from build123d import *

# Parameters (mm, degrees)
BOSS_EXTRUDE3_DEPTH = 12
BOSS_EXTRUDE4_DEPTH = 20
BOSS_EXTRUDE5_DEPTH = 12
SKETCH12_W          = 16
SKETCH12_H          = 40
CUT_EXTRUDE1_DEPTH  = 96.833188406
SKETCH13_R          = 8
CUT_EXTRUDE2_DEPTH  = 94.808315196
SKETCH14_R          = 8
CUT_EXTRUDE3_DEPTH  = 96.833188406
SKETCH15_R          = 8
CUT_EXTRUDE4_DEPTH  = 119.321595662
FILLET1_R           = 3
FILLET2_R           = 2


with BuildPart() as part:
    # Sketch7 → Boss-Extrude3 (new body)
    with BuildSketch(Plane(origin=(0, 0, 0), x_dir=(0, 1, 0), z_dir=(0, 0, 1))):
        with BuildLine():
            Line((0, -20), (0, 20))
            Line((0, 20), (40, 20))
            ThreePointArc((40, 20), (60, 0), (40, -20))
            Line((40, -20), (0, -20))
        make_face()
    extrude(amount=BOSS_EXTRUDE3_DEPTH)

    # Sketch9 → Boss-Extrude4 (add, symmetric)
    with BuildSketch(Plane.YZ):
        with BuildLine():
            Line((0, 0), (-40, 0))
            Line((-40, 0), (-40, 40))
            ThreePointArc((-40, 40), (-20, 60), (0, 40))
            Line((0, 40), (0, 0))
        make_face()
    extrude(amount=BOSS_EXTRUDE4_DEPTH, both=True)

    # Sketch10 → Boss-Extrude5 (add)
    with BuildSketch(Plane.XZ.offset(40)):
        with BuildLine():
            Line((-20, 0), (20, 0))
            Line((20, 0), (20, -39.999997874))
            ThreePointArc((20, -39.999997874), (1.063e-06, -60), (-20, -40))
            Line((-20, -40), (-20, 0))
        make_face()
    extrude(amount=-BOSS_EXTRUDE5_DEPTH)

    # Sketch12 → Cut-Extrude1 (cut, through all)
    with BuildSketch(Plane.XY.offset(12)):
        with Locations((0, -20)):
            Rectangle(SKETCH12_W, SKETCH12_H)
    extrude(amount=CUT_EXTRUDE1_DEPTH, mode=Mode.SUBTRACT)

    # Sketch13 → Cut-Extrude2 (cut, through all)
    with BuildSketch(Plane.YZ.offset(20)):
        with Locations((-20, 40)):
            Circle(SKETCH13_R)
    extrude(amount=-CUT_EXTRUDE2_DEPTH, mode=Mode.SUBTRACT)

    # Sketch14 → Cut-Extrude3 (cut, through all)
    with BuildSketch(Plane.XY.offset(12)):
        with Locations((0, 40)):
            Circle(SKETCH14_R)
    extrude(amount=-CUT_EXTRUDE3_DEPTH, mode=Mode.SUBTRACT)

    # Sketch15 → Cut-Extrude4 (cut, through all)
    with BuildSketch(Plane.XZ.offset(40)):
        with Locations(Location((0, -40, 0), (0, 0, 270))):
            Circle(SKETCH15_R)
    extrude(amount=-CUT_EXTRUDE4_DEPTH, mode=Mode.SUBTRACT)

    # Fillet1
    fillet1_edges = [part.edges().sort_by_distance(p)[0] for p in [
        (14, 0, 12),
        (-14, 0, 12),
    ]]
    fillet(fillet1_edges, radius=FILLET1_R)

    # Fillet2
    fillet2_edges = [part.edges().sort_by_distance(p)[0] for p in [
        (0, -28, 0),
    ]]
    fillet(fillet2_edges, radius=FILLET2_R)


solid = part.part
Here's how the part is built. I have some questions about the finished solid (model axes, mm). A direction names the side the tool comes from. Round coordinates to 2 decimals unless told otherwise and drop trailing zeros. Order: outer loops, then holes, each group sorted by start corner. A loop starts at its lowest first (then second) coordinate and runs counter-clockwise, first axis right, second up. Notation, with made-up numbers: (-17.75, -2.75) -> (41.25, -2.75) arc R22 cw to (41.25, 8.25) -> close; hole circle Ø3 at (27.5, 8.25). An arc over 180 degrees is marked (long way). Return JSON: item names as keys, results as strings.
Q1. For pin 1 Ø20 at (x, y) = (-7.5, 6) entering from +Z; pin 2 Ø1 at (x, y) = (10.5, 40.5) entering from -Z; pin 3 Ø1.5 at (x, z) = (0.5, -47) entering from +Y; pin 4 Ø1.5 at (x, z) = (-6.5, -36) entering from +Y, each with a flat end and sliding along its axis, tell me the tip position at first contact or that it passes through.
Filled sheet:
{"pin 1": "stops at z = 51.98", "pin 2": "stops at z = 0", "pin 3": "passes through", "pin 4": "stops at y = -28"}
Q2. I need wall thicknesses on line 1 along Z through (x, y) = (14, -20); line 2 along Z through (x, y) = (14.5, 31.5); line 3 along Y through (x, z) = (-18, 23). Which ranges of each line are inside material? Lowest first, please. Write a range as from..to.
Filled sheet:
{"line 1": "z = 0..32, 48..60", "line 2": "z = 0..12", "line 3": "y = -40..0"}
Q3. If we section it at D-D on z = 37: List the corners of the cut face in (x, y) for me.
Filled sheet:
{"outline": "(-20, -40) -> (-8, -40) -> (-8, -27.42) -> (-20, -27.42) -> close; (-20, -12.58) -> (-8, -12.58) -> (-8, 0) -> (-20, 0) -> close; (8, -40) -> (20, -40) -> (20, -27.42) -> (8, -27.42) -> close; (8, -12.58) -> (20, -12.58) -> (20, 0) -> (8, 0) -> close"}
Q4. If we section it at C-C on y = -20: List the corners of the cut face in (x, z) for me, plus the area to 3 significant figures.
Filled sheet:
{"outline": "(-20, 0) -> (20, 0) -> (20, 32) -> (8, 32) -> (8, 12) -> (-8, 12) -> (-8, 32) -> (-20, 32) -> close; (-20, 48) -> (-8, 48) -> (-8, 60) -> (-20, 60) -> close; (8, 48) -> (20, 48) -> (20, 60) -> (8, 60) -> close", "area": "1,250 mm^2"}
Q5. If we section it at B-B on z = 22.5: List the corners of the cut face in (x, y) for me, plus the area to 3 significant figures.
Filled sheet:
{"outline": "(-20, -40) -> (-8, -40) -> (-8, 0) -> (-20, 0) -> close; (8, -40) -> (20, -40) -> (20, 0) -> (8, 0) -> close", "area": "960 mm^2"}
Q6. If we section it at A-A on x = 0: List the corners of the cut face in (y, z) for me.
Filled sheet:
{"outline": "(-40, -60) -> (-28, -60) -> (-28, -48) -> (-40, -48) -> close; (-40, -32) -> (-28, -32) -> (-28, -2) arc R2 cw to (-26, 0) -> (32, 0) -> (32, 12) -> (-40, 12) -> close; (48, 0) -> (60, 0) -> (60, 12) -> (48, 12) -> close"}
Q7. If we mould it in two halves opening along X, with no side actions, what happens to faces 5 (the cylindrical face through (-4.868, -34.084, -33.651)), 6 (the cylindrical face through (0, -34, -60)), 7 (the cylindrical face through (-13.916, -21.041, 47.932))? For each: released by +X, released by -X, zero draft, split by the parting line, or undercut.
Filled sheet:
{"face 5": "undercut", "face 6": "split by the parting line", "face 7": "zero draft"}
Q8. Which directions (+Z, -Z, +X, -X, +Y, -Y) give clear straight access to the entire face, cutting with the end or side of a thin tool? Please do faces 1 (the cylindrical face through (14, -20, 60)), 2 (the flat face through (14, 0, 28)), 3 (the flat face through (-8, -19, 30)), 4 (the flat face through (0, 18, 0)).
Filled sheet:
{"face 1": "+Z, +X, -X", "face 2": "+Z, +X, -X, +Y", "face 3": "+Z, +Y, -Y", "face 4": "-Z, +X, -X, +Y"}
